Model file for the job. Use its own axes, mm. Face numbers are marked on the shaded views. Give positions to 0.01 mm unless a question says otherwise; leave off trailing zeros. Loops run counter-clockwise (first coordinate to the right, second up) from the corner with the lowest first, then second, coordinate; pieces in that order, holes last. Notation, with made-up numbers: (46, -37) - (99, -37) arc R25 ccw to (99, -20) - close; hole circle Ø5 at (-29.5, 87.25). An arc over 180 degrees is marked (long way). Answer as CSV lines item,"result". Start each with the question number.
Item 1: Saw through at D-D on y = 113. Give the cut face in (x, z), plus the area to 3 significant figures.
Item 2: Saw through at A-A on y = 134. Give the cut face in (x, z), plus the area to 3 significant figures.
Item 3: Pin check, flat tips, straight feed: pin 1 (1 mm diameter, centred on x = 104, z = 45.5, fed in from +Y); pin 2 (12 mm diameter, centred on x = 74, z = 90.5, fed in from +Y). Stop position of each tip, or through.
Item 4: Drill centre lines: L1, parallel to X at y = 119, z = 42; L2, parallel to X at y = 144.5, z = 64; L3, parallel to Y at x = 101.5, z = 14.5. Where is each one in solid material? Low to high. Write a range as from..to.
Item 5: Saw through at C-C on x = 92. Give the cut face in (y, z).
Item 6: Saw through at B-B on z = 10. Give the cut face in (x, y), plus the area to 3 significant figures.
Item 7: Pull direction X, two halves, no side cores. Call the marked faces 1, 2, 3 and 4: pulls with the +X half, pulls with the -X half, needs draft (parallel to the pull), parting line crosses it, or undercut.
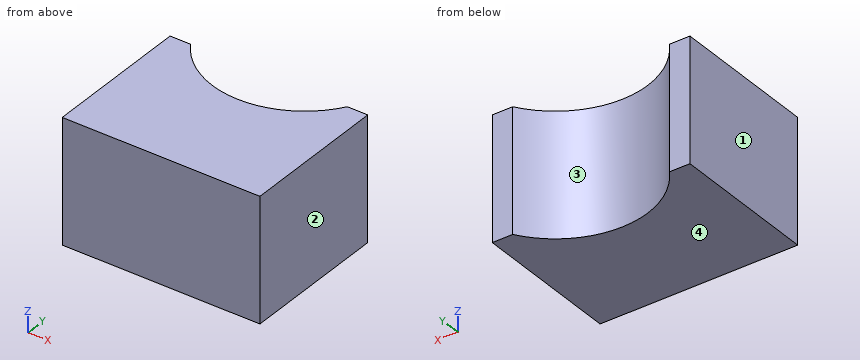
Autodesk Inventor part; units mm, degrees
ref_plane "YZ Plane" through (0, 0, 0) normal (1, 0, 0) x (0, 1, 0)
ref_plane "XZ Plane" through (0, 0, 0) normal (0, 1, 0) x (-1, 0, 0)
ref_plane "XY Plane" through (0, 0, 0) normal (0, 0, 1) x (1, 0, 0)
sketch "Sketch1" plane through (0, 0, 0) normal (0, 0, 1) x (1, 0, 0)
  line L0 (0, 0) -> (203.2, 0)
  line L1 (203.2, 0) -> (203.2, 152.4)
  line L2 (0, 152.4) -> (0, 0)
  line L3 (203.2, 152.4) -> (196.85, 152.4)
  line L4 (6.35, 152.4) -> (0, 152.4)
  line L5 (101.6, 152.4) -> (101.6, 203.2)
  arc A0 (21.0275, 152.4) -> (182.1725, 152.4) centre (101.6, 203.2) ccw
  line L6 (6.35, 152.4) -> (21.0275, 152.4)
  line L7 (182.1725, 152.4) -> (196.85, 152.4)
  dimension "d0" = 203.2
  dimension "d1" = 152.4
  dimension "d5" = 50.8
  dimension "d6" = 190.5
extrude "Extrusion1" add sketch "Sketch1" along normal blind 127
properties part number "tankMount"
Responses:
1,outline,"(0, 0) - (71, 0) - (71, 127) - (0, 127) - close; (132.2, 0) - (203.2, 0) - (203.2, 127) - (132.2, 127) - close"
1,area,"18,000 mm2"
2,outline,"(0, 0) - (36.15, 0) - (36.15, 127) - (0, 127) - close; (167.05, 0) - (203.2, 0) - (203.2, 127) - (167.05, 127) - close"
2,area,"9,180 mm2"
3,pin 1,"y = 107.99"
3,pin 2,"y = 114.07"
4,L1,"0..57.07, 146.13..203.2"
4,L2,"0..26.59, 176.61..203.2"
4,L3,"0..107.95"
5,outline,"(0, 0) - (108.43, 0) - (108.43, 127) - (0, 127) - close"
6,outline,"(0, 0) - (203.2, 0) - (203.2, 152.4) - (182.17, 152.4) arc R95.25 cw to (21.03, 152.4) - (0, 152.4) - close"
6,area,"25,900 mm2"
7,face 1,"pulls with the -X half"
7,face 2,"pulls with the +X half"
7,face 3,"undercut"
7,face 4,"needs draft"
